Geometry: see drawing. Coordinates: mm, zero at the bounding-box minimum. Coordinates: 2 decimals unless noted, no trailing zeros. Order: outer loops, then holes, each group sorted by start corner. A loop starts at its lowest first (then second) coordinate and runs counter-clockwise, first axis right, second up.
Item 1: Section D-D on x = 28.5. Return the cut outline in (y, z).
Item 2: Ray query, line 1 (X direction, y = 8.75, z = 3.05); line 2 (Z direction, x = 30, y = 9.75); line 3 (X direction, y = 14.25, z = 3.45). Return the intervals inside material, ascending.
Item 3: Section A-A on x = 3. Return the cut outline in (y, z), then the cut area to 3 significant figures.
Item 4: Mould query, pull axis X, two halves, no side actions, for the marked faces 1, 2 and 3. Classes: released by +X, released by -X, zero draft, split by the parting line, or undercut.
Item 5: Section B-B on z = 3. Return the cut outline in (x, y), then the cut area to 3 significant figures.
Item 6: Section C-C on y = 7.5. Return the cut outline in (x, z).
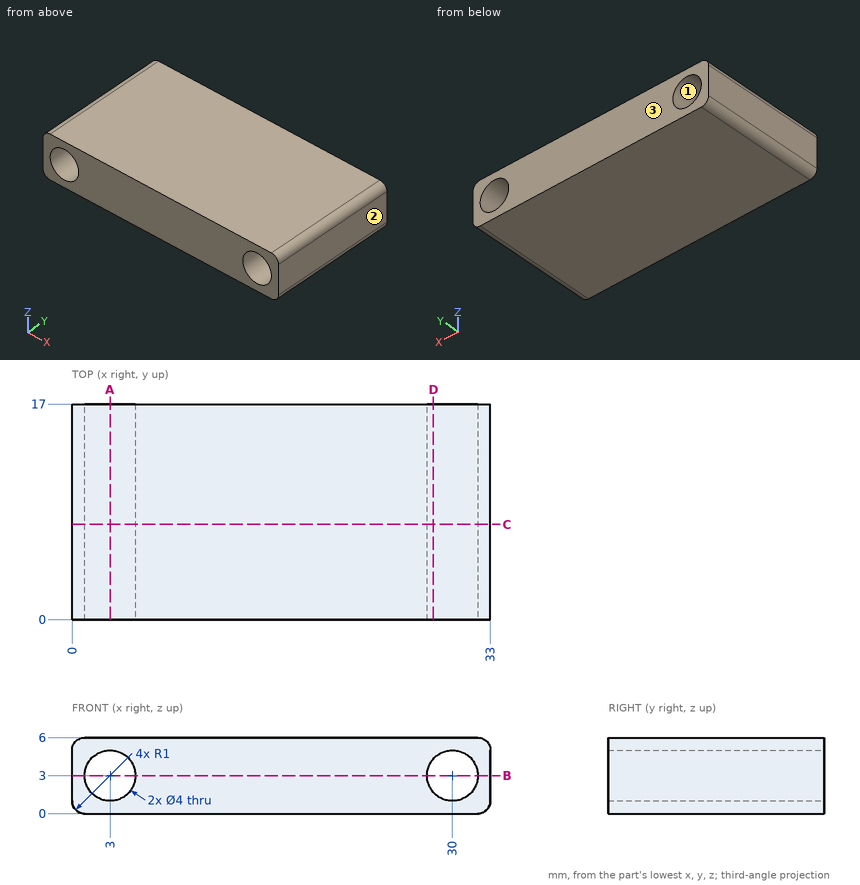
Answer list:
1. outline: (0, 0) - (17, 0) - (17, 1.68) - (0, 1.68) - close; (0, 4.32) - (17, 4.32) - (17, 6) - (0, 6) - close
2. line 1: x = 0 to 1, 5 to 28, 32 to 33
2. line 2: z = 0 to 1, 5 to 6
2. line 3: x = 0 to 1.05, 4.95 to 28.05, 31.95 to 33
3. outline: (0, 0) - (17, 0) - (17, 1) - (0, 1) - close; (0, 5) - (17, 5) - (17, 6) - (0, 6) - close
3. area: 34.0 mm2
4. face 1: undercut
4. face 2: released by +X
4. face 3: zero draft
5. outline: (0, 0) - (1, 0) - (1, 17) - (0, 17) - close; (5, 0) - (28, 0) - (28, 17) - (5, 17) - close; (32, 0) - (33, 0) - (33, 17) - (32, 17) - close
5. area: 425 mm2
6. outline: (0, 1) arc R1 ccw to (1, 0) - (32, 0) arc R1 ccw to (33, 1) - (33, 5) arc R1 ccw to (32, 6) - (1, 6) arc R1 ccw to (0, 5) - close; hole circle Ø4 at (3, 3); hole circle Ø4 at (30, 3)
